Geometry: final body of the model. Coordinates: model frame, mm. A direction names the side the tool comes from. Round coordinates to 2 decimals unless told otherwise and drop trailing zeros. Write each loop counter-clockwise with the first axis right and the second up, starting at its lowest first coordinate (ties: lowest second). Pieces come first, ordered by that corner, then holes. Notation, with made-up numbers: M -3,-38.75 L 50,-38.75 A20 cw 50,-10.75 Z; hole C 10,77 d1. An arc over 180 degrees is marked long. Use one line per item in the form item = value. Start each with the question number.
Item 1: Ray query, probe 1 along X at (y, z) = (2.2, 1); probe 2 along X at (y, z) = (0.5, 4.75); probe 3 along Z at (x, y) = (16.5, 2.1). Return the intervals inside material, ascending.
Item 2: Section query A-A (z = 6.75). Return loops of the section in (x, y), and give its area (3 significant figures).
Item 3: Section query B-B (y = 0.8). Return loops of the section in (x, z), and give its area (3 significant figures).
Item 4: Pull-direction query (Z, two-part tool) for faces 6 (the flat face through (37, 0, 0)), 7 (the flat face through (66, 1, 4)), 8 (the flat face through (15, 2, 6)); classes: pulls with the +Z half, pulls with the -Z half, needs draft (parallel to the pull), parting line crosses it, or undercut.
Item 5: Section query C-C (z = 1.5). Return loops of the section in (x, y), and give its area (3 significant figures).
Item 6: Reachability of faces 1 (the flat face through (6, 1, 0)), 2 (the flat face through (36, 1, 2)), 3 (the flat face through (42, 1, 4)), 4 (the flat face through (36, 1, -4)), 5 (the flat face through (18, 2, 8)) from +Z, -Z, +X, -X, +Y, -Y: full face, straight path, thin tool, end or side. Return the list, or none.
Item 7: Pin query (flat end, axial travel): pin 1 Ø1.5 at (y, z) = (1.5, 1) entering from -X; pin 2 Ø0.9 at (x, y) = (44, 1.5) entering from +Z; pin 3 Ø1.5 at (y, z) = (1, 6) entering from +X. Return the tip coordinate at first contact, or that it passes through.
Item 8: Section query D-D (x = 51). Return loops of the section in (y, z).
Autodesk Inventor part; units mm, degrees
ref_plane "YZ Plane" through (0, 0, 0) normal (1, 0, 0) x (0, 1, 0)
ref_plane "XZ Plane" through (0, 0, 0) normal (0, 1, 0) x (-1, 0, 0)
ref_plane "XY Plane" through (0, 0, 0) normal (0, 0, 1) x (1, 0, 0)
sketch "Эскиз1" plane through (0, 0, 0) normal (0, 1, 0) x (-1, 0, 0)
  line L0 (-4, -4) -> (-68, -4)
  line L1 (-72, 0) -> (-72, 4)
  line L2 (0, 0) -> (-3.643, -3.643)
  line L3 (-3.643, -3.643) -> (-4, -4)
  line L4 (-48, 4) -> (-48, 0)
  line L5 (-48, 4) -> (-48, 0)
  line L6 (-36, 4) -> (-36, 0)
  line L7 (-60, 4) -> (-60, 0)
  line L8 (-72, 4) -> (-60, 4)
  line L9 (-48, 4) -> (-36, 4)
  line L10 (-60, 0) -> (-48, 0)
  line L11 (-36, 0) -> (-24, 0)
  line L12 (-12, 0) -> (0, 0)
  line L13 (-68, -4) -> (-72, 0)
  line L14 (-24, 11) -> (-12, 11)
  line L15 (-12, 11) -> (-12, 0)
  line L16 (-24, 11) -> (-24, 0)
  point P0 (0, 0)
  point P1 (-48, 2)
  point P2 (-72, 2)
  point P3 (-48, 2)
  point P4 (-12, 2)
  point P5 (-36, 2)
  point P6 (-60, 2)
  point P7 (-30, 0)
  point P8 (-3.8215, -3.8215)
  dimension "d9" = 24
  dimension "d13" = 12
  dimension "d19" = 4
  dimension "d23" = 8
  dimension "d26" = 135
  dimension "d28" = 72
  dimension "d29" = 12
  dimension "d30" = 11
extrude "Выдавливание1" add sketch "Эскиз1" along normal blind 3
sketch "Эскиз2" plane through (0, 3, 0) normal (0, 1, 0) x (1, 0, 0)
  line L0 (12, 0) -> (12, -11) construction
  line L1 (12, -11) -> (24, -11) construction
  line L2 (15, -4) -> (15, -8)
  line L3 (15, -8) -> (21, -8)
  line L4 (15, -4) -> (21, -4)
  line L5 (21, -4) -> (21, -8)
  line L6 (24, -11) -> (24, 0)
  point P0 (0, 0)
  point P1 (21, -6)
  dimension "d31" = 3
  dimension "d32" = 4
  dimension "d33" = 3
  dimension "d36" = 3
extrude "Выдавливание2" cut sketch "Эскиз2" against normal blind 10
properties part number "креп"
Working result:
q1.probe_1 = 12 to 24, 36 to 48, 60 to 72
q1.probe_2 = 12 to 15, 21 to 24
q1.probe_3 = -4 to 4, 8 to 11
q2.outline = M 12,0 L 15,0 L 15,3 L 12,3 Z; M 21,0 L 24,0 L 24,3 L 21,3 Z
q2.area = 18.0 mm²
q3.outline = M 0,0 L 4,-4 L 68,-4 L 72,0 L 72,4 L 60,4 L 60,0 L 48,0 L 48,4 L 36,4 L 36,0 L 24,0 L 24,11 L 12,11 L 12,0 Z; hole M 15,4 L 21,4 L 21,8 L 15,8 Z
q3.area = 476 mm²
q4.face_6 = needs draft
q4.face_7 = pulls with the +Z half
q4.face_8 = undercut
q5.outline = M 12,0 L 24,0 L 24,3 L 12,3 Z; M 36,0 L 48,0 L 48,3 L 36,3 Z; M 60,0 L 72,0 L 72,3 L 60,3 Z
q5.area = 108 mm²
q6.face_1 = +Z, -X, +Y, -Y
q6.face_2 = +Z, +Y, -Y
q6.face_3 = +Z, +X, +Y, -Y
q6.face_4 = -Z, +X, -X, +Y, -Y
q6.face_5 = +Y, -Y
q7.pin_1 = 12
q7.pin_2 = 4
q7.pin_3 = 24
q8.outline = M 0,-4 L 3,-4 L 3,0 L 0,0 Z
